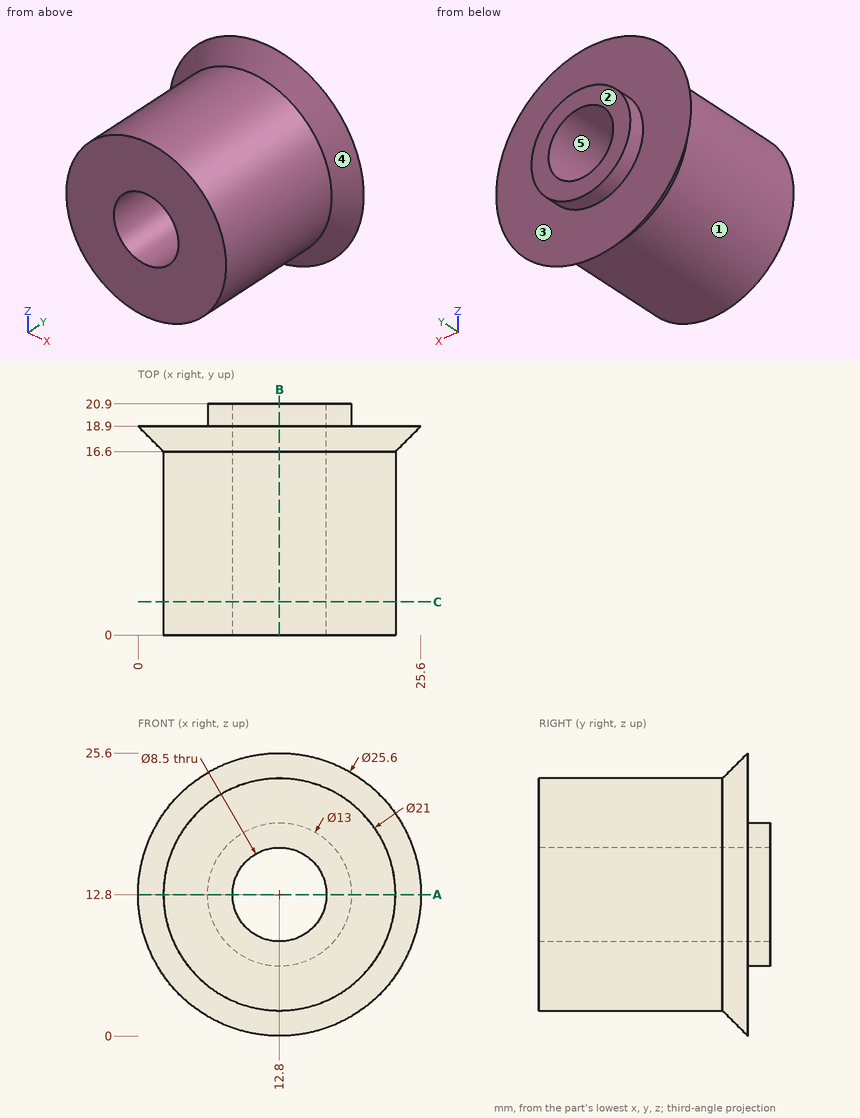
Check sheet for the drawn part. Datum: minimum x, y, z corner. Units: mm. A direction names the side the tool comes from. Round coordinates to 2 decimals unless told otherwise and drop trailing zeros. Loops run counter-clockwise (first coordinate to the right, second up) from the corner with the lowest first, then second, coordinate; pieces in that order, holes last. Notation, with made-up numbers: M 13,-7.75 L 43,-7.75 A17 ccw 43,21.25 Z; hole C 46,-6 d1. An arc over 180 degrees is marked long. One line per question, with ' | ' between items. Start each with the question number.
Item 1: Scan lines: probe 1 along X at (y, z) = (8.75, 12.8); probe 2 along Y at (x, z) = (10, 19.25); probe 3 along X at (y, z) = (6.75, 11). Record each from-to range of solid material in increasing order.
Item 2: Release check for a two-part mould opening along Z. For the marked faces 3, 4 and 5 record: released by +Z, released by -Z, zero draft, split by the parting line, or undercut.
Item 3: Section check A-A (z = 12.8). Record the boundary of the cut face in (x, y).
Item 4: Section check C-C (y = 3). Record the boundary of the cut face in (x, z), and give its area (3 significant figures).
Item 5: Gauge pin test, flat ends, axial feed: pin 1 Ø5 at (x, z) = (22, 6) entering from +Y; pin 2 Ø6 at (y, z) = (11, 7) entering from +X; pin 3 Ø4 at (x, y) = (2.5, 4) entering from +Z. Record the tip position at first contact, or that the pin passes through.
Item 6: Section check B-B (x = 12.8). Record the boundary of the cut face in (y, z), and give its area (3 significant figures).
Item 7: Set-up check for the marked faces 1 and 2: record each of +Z, -Z, +X, -X, +Y, -Y from which the full face is reachable in a straight line by a thin tool's end or side.
Worked out:
1) probe 1: 2.3 to 8.55, 17.05 to 23.3 | probe 2: 0 to 18.9 | probe 3: 2.46 to 8.95, 16.65 to 23.14
2) face 3: zero draft | face 4: split by the parting line | face 5: undercut
3) outline: M 0,18.9 L 2.3,16.6 L 2.3,0 L 8.55,0 L 8.55,20.9 L 6.3,20.9 L 6.3,18.9 Z; M 17.05,0 L 23.3,0 L 23.3,16.6 L 25.6,18.9 L 19.3,18.9 L 19.3,20.9 L 17.05,20.9 Z
4) outline: C 12.8,12.8 d21; hole C 12.8,12.8 d8.5 | area: 290 mm^2
5) pin 1: y = 18.9 | pin 2: x = 22.92 | pin 3: z = 19.23
6) outline: M 0,2.3 L 16.6,2.3 L 18.9,0 L 18.9,6.3 L 20.9,6.3 L 20.9,8.55 L 0,8.55 Z; M 0,17.05 L 20.9,17.05 L 20.9,19.3 L 18.9,19.3 L 18.9,25.6 L 16.6,23.3 L 0,23.3 Z | area: 251 mm^2
7) face 1: -Y | face 2: +Z, -Z, +X, -X, +Y
